```python
from build123d import *

# Parameters (mm, degrees)
F0_W     = 101.6
F0_H     = 1524
F1_DEPTH = 50.8
F3_DEPTH = 50.8
F5_DEPTH = 50.8


with BuildPart() as f1:
    # F0 (on Front) → F1 (new body)
    with BuildSketch(Plane.XZ):
        with Locations((50.8, 762)):
            Rectangle(F0_W, F0_H)
    extrude(amount=F1_DEPTH)

    # F2 (on Front) → F3 (join)
    with BuildSketch(Plane.XZ):
        Polygon((0, 1524), (-863.6, 101.6), (-744.7400515441, 101.6), (0, 1328.2306731315), align=None)
        Polygon((-863.6, 0), (0, 0), (0, 101.6), (-744.7400515441, 101.6), (-863.6, 101.6), align=None)
        Polygon((101.6, 101.6), (101.6, 0), (965.2, 0), (965.2, 101.6), (846.3400515441, 101.6), align=None)
        Polygon((846.3400515441, 101.6), (965.2, 101.6), (101.6, 1524), (101.6, 1328.2306731315), align=None)
    extrude(amount=F3_DEPTH)

    # F4 (on Front) → F5 (join)
    with BuildSketch(Plane.XZ):
        Polygon((-343.782908687, 762), (0, 762), (0, 863.6), (-282.0971944012, 863.6), align=None)
        Polygon((383.6971944012, 863.6), (101.6, 863.6), (101.6, 762), (445.382908687, 762), align=None)
    extrude(amount=F5_DEPTH)


solid = f1.part
```
The model under review builds one solid part; all positions refer to its coordinate system, in mm. A direction names the side the tool comes from. Round coordinates to 2 decimals unless told otherwise and drop trailing zeros. Order: outer loops, then holes, each group sorted by start corner. A loop starts at its lowest first (then second) coordinate and runs counter-clockwise, first axis right, second up.
Item 1: Draft analysis for pull direction X (two halves, no side actions). For faces 3 (the flat face through (0, -25, 427)), 4 (the flat face through (50, -25, 1524)), 5 (the flat face through (-425.755, -25.044, 822.757)), state which applies: released by +X, released by -X, zero draft, split by the parting line, or undercut.
Working result:
face 3: undercut
face 4: zero draft
face 5: released by -X
Item 2: Add section B-B, the plane x = -447. State the section outline as (y, z) points, and give its area (3 significant figures).
Working result:
outline: (-50.8, 0) - (0, 0) - (0, 101.6) - (-50.8, 101.6) - close; (-50.8, 592) - (0, 592) - (0, 787.76) - (-50.8, 787.76) - close
area: 15,100 mm2
Item 3: Add section D-D, the plane z = 464. State the section outline as (x, y) points, and give its area (3 significant figures).
Working result:
outline: (-643.57, -50.8) - (-524.71, -50.8) - (-524.71, 0) - (-643.57, 0) - close; (0, -50.8) - (101.6, -50.8) - (101.6, 0) - (0, 0) - close; (626.31, -50.8) - (745.17, -50.8) - (745.17, 0) - (626.31, 0) - close
area: 17,200 mm2
Item 4: Add section A-A, the plane y = -40. State the section outline as (x, z) points.
Working result:
outline: (-863.6, 0) - (965.2, 0) - (965.2, 101.6) - (101.6, 1524) - (0, 1524) - (-863.6, 101.6) - close; hole (-744.74, 101.6) - (0, 101.6) - (0, 762) - (-343.78, 762) - close; hole (-282.1, 863.6) - (0, 863.6) - (0, 1328.23) - close; hole (101.6, 101.6) - (846.34, 101.6) - (445.38, 762) - (101.6, 762) - close; hole (101.6, 863.6) - (383.7, 863.6) - (101.6, 1328.23) - close
Item 5: Machinability: for faces 1 (the flat face through (539.445, -25.044, 802.843)), 2 (the flat face through (-367, -25, 101.6)), which of the approach directions +Z, -Z, +X, -X, +Y, -Y give a long, thin tool a straight path to every point of the face, cutting with its end or side? Answer none if there is none.
Working result:
face 1: +Z, +X, +Y, -Y
face 2: +Y, -Y
Item 6: To check wall thickness, follow probe 1 along Z at (x, y) = (-56, -18); probe 2 along Z at (x, y) = (182, -3); probe 3 along X at (y, z) = (-9, 582). State the ranges of each line that lie inside material, in increasing order.
Working result:
probe 1: z = 0 to 101.6, 762 to 863.6, 1236 to 1431.76
probe 2: z = 0 to 101.6, 762 to 863.6, 1195.81 to 1391.58
probe 3: x = -571.93 to -453.07, 0 to 101.6, 554.67 to 673.53
Item 7: Add section C-C, the plane x = -198.5. State the section outline as (y, z) points, and give its area (3 significant figures).
Working result:
outline: (-50.8, 0) - (0, 0) - (0, 101.6) - (-50.8, 101.6) - close; (-50.8, 762) - (0, 762) - (0, 863.6) - (-50.8, 863.6) - close; (-50.8, 1001.29) - (0, 1001.29) - (0, 1197.06) - (-50.8, 1197.06) - close
area: 20,300 mm2
Item 8: For pin 1 (4 mm diameter, centred on y = -37, z = 432, fed in from +X); pin 2 (6 mm diameter, centred on y = -7, z = 1008.5, fed in from +X); pin 3 (15 mm diameter, centred on x = 546, y = -36.5, fed in from +Z), all flat-tipped, find the tip position at first contact; note any pin that passes through.
Working result:
pin 1: stops at x = 765.81
pin 2: stops at x = 416.4
pin 3: stops at z = 804.4
